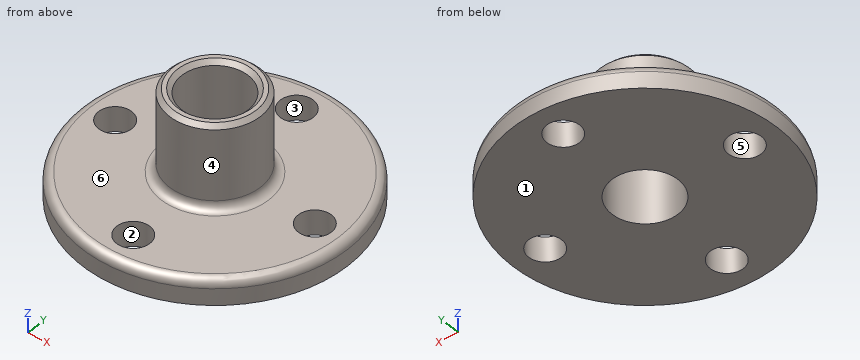
Autodesk Inventor part; units mm, degrees
ref_plane "YZ Plane" through (0, 0, 0) normal (1, 0, 0) x (0, 1, 0)
ref_plane "XZ Plane" through (0, 0, 0) normal (0, 1, 0) x (-1, 0, 0)
ref_plane "XY Plane" through (0, 0, 0) normal (0, 0, 1) x (1, 0, 0)
sketch "Эскиз1" plane through (0, 0, 0) normal (0, 0, 1) x (1, 0, 0)
  circle A0 centre (0, 0) radius 16
  circle A1 centre (0, 0) radius 12
  circle A2 centre (-12, 0) radius 2
  circle A3 centre (0, -12) radius 2
  circle A4 centre (12, 0) radius 2
  circle A5 centre (0, 12) radius 2
  circle A6 centre (0, 0) radius 4
  dimension "d1" = 24
  dimension "d0" = 32
  dimension "d2" = 4
  dimension "d5" = 360
  dimension "d7" = 8
extrude "Выдавливание1" add sketch "Эскиз1" along normal blind 3 contours A0 | A4 A1 A3 A2 A5
sketch "Эскиз2" plane through (0, 0, 3) normal (0, 0, 1) x (1, 0, 0)
  circle A0 centre (0, 0) radius 5.5
  circle A1 centre (0, 0) radius 16
  circle A2 centre (0, 12) radius 2
  circle A3 centre (-12, 0) radius 2
  circle A4 centre (0, -12) radius 2
  circle A5 centre (0, 0) radius 4
  circle A6 centre (12, 0) radius 2
  dimension "d10" = 11
extrude "Выдавливание2" add sketch "Эскиз2" along normal blind 10 contours A0
fillet "Сопряжение1" radius 1 2 edges at (-16, 0, 3) (-5.5, 0, 3)
chamfer "Фаска1" distance 0.5 angle 45 2 edges at (-5.5, 0, 13) (-4, 0, 13)
properties part number "МУФТА НА ВАЛ бол"
For this review, take the finished solid that the model builds, in its own axes (mm). Face numbers are marked on the shaded views. A direction names the side the tool comes from. Round coordinates to 2 decimals unless told otherwise and drop trailing zeros. Write each loop counter-clockwise with the first axis right and the second up, starting at its lowest first coordinate (ties: lowest second). Pieces come first, ordered by that corner, then holes. Notation, with made-up numbers: (-13, 6.5) - (8, 6.5) arc R25 ccw to (8, 43.5) - close; hole circle Ø5 at (57.5, -22.75). An arc over 180 degrees is marked (long way). Write item = value, one per line. Start each with the question number.
1. For pin 1 Ø6 at (x, z) = (5, 8.5) entering from -Y; pin 2 Ø6.5 at (x, y) = (12, 0) entering from +Z; pin 3 Ø3.5 at (x, y) = (-12, 0) entering from +Z; pin 4 Ø5 at (x, z) = (6, 5) entering from -Y, all flat-tipped, find the tip position at first contact; note any pin that passes through.
2. For the marked faces 5 and 6, list the 3-axis set-ups (+Z, -Z, +X, -X, +Y, -Y) from which the entire face can be reached by the end or side of a thin tool; tool diameter is ignored.
3. Consider section A-A on y = 0. State the section outline as (x, z) points.
4. Consider section C-C on z = 7.5. State the section outline as (x, y) points, plus the area to 3 significant figures.
5. Draft analysis for pull direction Y (two halves, no side actions). For the marked faces 1, 2, 3 and 4, state which applies: released by +Y, released by -Y, zero draft, split by the parting line, or undercut.
6. Wall thickness on L1, parallel to Y at x = 0, z = 1.8; L2, parallel to Y at x = 0, z = 5; L3, parallel to X at y = 1.5, z = 1.75: over which ranges is each line inside the solid? List them lowest first.
Evaluation:
q1.pin_1 = -5.12
q1.pin_2 = 3
q1.pin_3 = through
q1.pin_4 = -14.9
q2.face_5 = +Z, -Z
q2.face_6 = +Z
q3.outline = (-16, 0) - (-14, 0) - (-14, 3) - (-15, 3) arc R1 ccw to (-16, 2) - close; (-10, 0) - (-4, 0) - (-4, 12.5) - (-4.5, 13) - (-5, 13) - (-5.5, 12.5) - (-5.5, 4) arc R1 cw to (-6.5, 3) - (-10, 3) - close; (4, 0) - (10, 0) - (10, 3) - (6.5, 3) arc R1 cw to (5.5, 4) - (5.5, 12.5) - (5, 13) - (4.5, 13) - (4, 12.5) - close; (14, 0) - (16, 0) - (16, 2) arc R1 ccw to (15, 3) - (14, 3) - close
q4.outline = circle Ø11 at (0, 0); hole circle Ø8 at (0, 0)
q4.area = 44.8 mm2
q5.face_1 = zero draft
q5.face_2 = undercut
q5.face_3 = undercut
q5.face_4 = split by the parting line
q6.L1 = -16 to -14, -10 to -4, 4 to 10, 14 to 16
q6.L2 = -5.5 to -4, 4 to 5.5
q6.L3 = -15.93 to -13.32, -10.68 to -3.71, 3.71 to 10.68, 13.32 to 15.93
